For this review, use the dimensioned drawing (mm, ordinates from the lowest corner) and the shaded views. Give positions to 0.01 mm unless a question says otherwise; leave off trailing zeros. Loops run counter-clockwise (first coordinate to the right, second up) from the corner with the lowest first, then second, coordinate; pieces in that order, holes last. Notation, with made-up numbers: (-13, -40) -> (7, -40) arc R22 cw to (7, -23) -> close; hole circle Ø9 at (39, 59). An arc over 180 degrees is marked (long way). Use a Markdown table: item, result. Add a question column.
1. For pin 1 Ø5 at (x, z) = (46, 4.5) entering from -Y, flat-tipped, find the tip position at first contact; note if it passes through.
2. Add section B-B (z = 9.75). State the section outline as (x, y) points.
3. Add section C-C (y = 2.15). Count the separate pieces of the cut face and the enclosed holes in it, and give its area (3 significant figures).
4. Add section D-D (x = 4). State the section outline as (y, z) points.
5. Add section A-A (x = 9.75). State the section outline as (y, z) points.
6. To check wall thickness, follow line 1 (Z direction, x = 40.25, y = 2.4); line 2 (Z direction, x = 17.5, y = 0.9); line 3 (X direction, y = 2.25, z = 19) (1 decimal). State the ranges of each line that lie inside material, in increasing order.
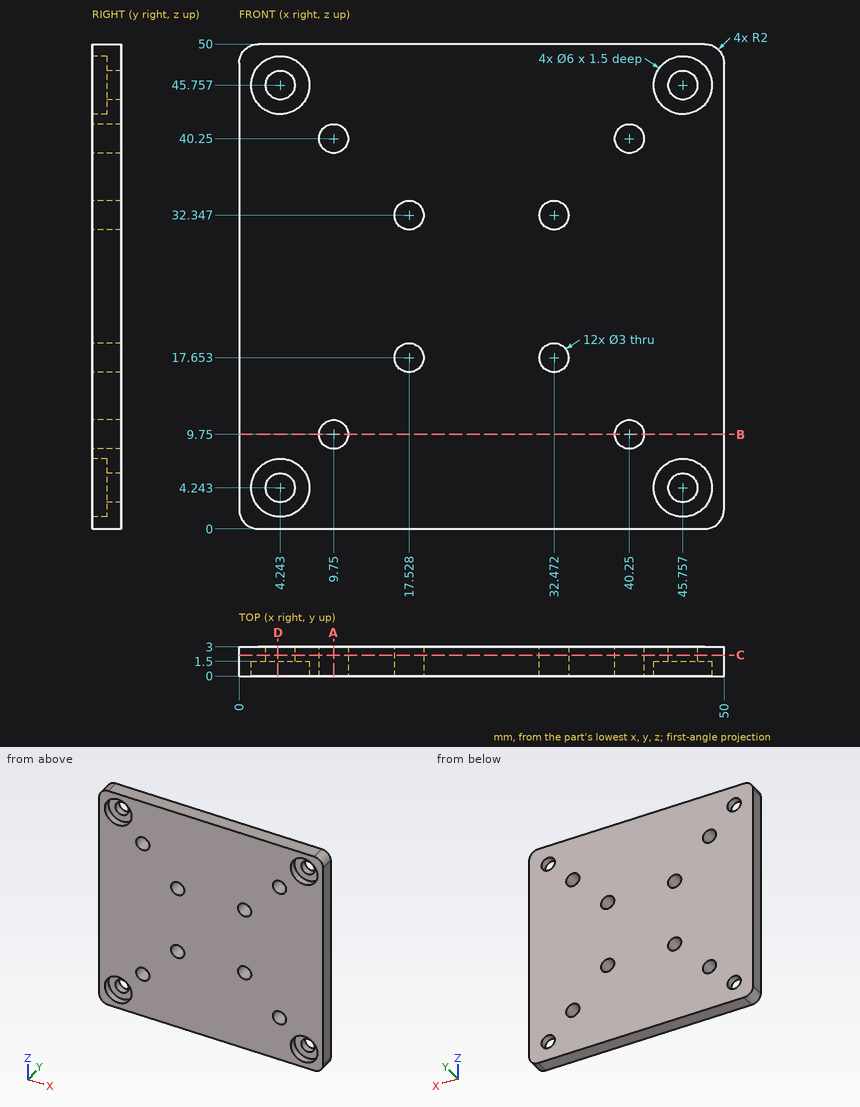
Taken from the geometry:
| question | item | result |
|---|---|---|
| 1 | pin 1 | stops at y = 1.5 |
| 2 | outline | (0, 0) -> (8.25, 0) -> (8.25, 3) -> (0, 3) -> close; (11.25, 0) -> (38.75, 0) -> (38.75, 3) -> (11.25, 3) -> close; (41.75, 0) -> (50, 0) -> (50, 3) -> (41.75, 3) -> close |
| 3 | separate pieces | 1 |
| 3 | enclosed holes | 12 |
| 3 | area | 2,410 mm^2 |
| 4 | outline | (0, 0) -> (3, 0) -> (3, 2.76) -> (1.5, 2.76) -> (1.5, 1.25) -> (0, 1.25) -> close; (0, 7.23) -> (1.5, 7.23) -> (1.5, 5.72) -> (3, 5.72) -> (3, 44.28) -> (1.5, 44.28) -> (1.5, 42.77) -> (0, 42.77) -> close; (0, 48.75) -> (1.5, 48.75) -> (1.5, 47.24) -> (3, 47.24) -> (3, 50) -> (0, 50) -> close |
| 5 | outline | (0, 0) -> (3, 0) -> (3, 8.25) -> (0, 8.25) -> close; (0, 11.25) -> (3, 11.25) -> (3, 38.75) -> (0, 38.75) -> close; (0, 41.75) -> (3, 41.75) -> (3, 50) -> (0, 50) -> close |
| 6 | line 1 | z = 0 to 8.25, 11.25 to 38.75, 41.75 to 50 |
| 6 | line 2 | z = 0 to 16.15, 19.15 to 30.85, 33.85 to 50 |
| 6 | line 3 | x = 0 to 16.9, 18.2 to 31.8, 33.1 to 50 |
